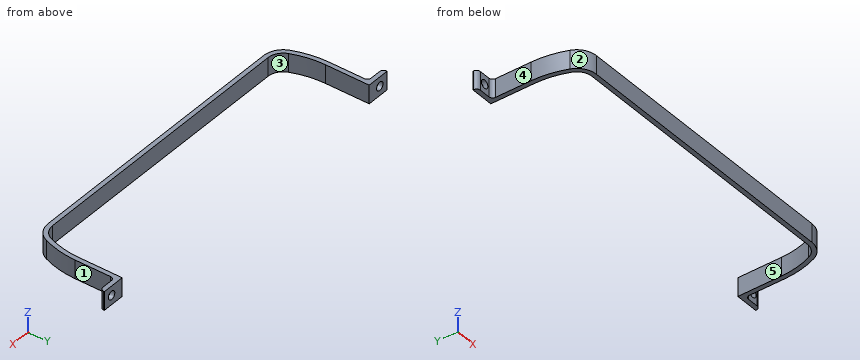
from build123d import *

# Parameters (mm, degrees)
F1_DEPTH = 5
F3_D     = 4.4958
F4_R     = 2


with BuildPart() as f1:
    # F0 (on Top) → F1 (new body, symmetric)
    with BuildSketch(Plane.XY):
        with BuildLine():
            Line((0, 2.4), (0, 0))
            Line((0, 0), (75, 0))
            ThreePointArc((75, 0), (80.9415780593, 1.816522709), (84.8515829028, 6.6449765723))
            ThreePointArc((84.8515829028, 6.6449765723), (87.5046708667, 15.6016514337), (88.4, 24.9))
            Line((88.4, 24.9), (88.4, 46))
            Line((88.4, 46), (98.4, 46))
            Line((98.4, 46), (98.4, 48.4))
            Line((98.4, 48.4), (86, 48.4))
            Line((86, 48.4), (86, 24.9))
            ThreePointArc((86, 24.9), (85.1487656265, 16.0595930226), (82.6263416519, 7.5440323965))
            ThreePointArc((82.6263416519, 7.5440323965), (79.5995150909, 3.8062128831), (75, 2.4))
            Line((75, 2.4), (0, 2.4))
        make_face()
    extrude(amount=F1_DEPTH, both=True)

    # F3 (through all)
    with Locations(Plane.XZ.offset(-46)):
        with Locations((93.4, 0)):
            Hole(F3_D / 2)

    # F4
    f4_edges = [f1.edges().sort_by_distance(p)[0] for p in [
        (88.4, 46, 0),
        (98.4, 46, 0),
    ]]
    fillet(f4_edges, radius=F4_R)

    # F5: F1 across face


with BuildPart() as f1_1:
    add(f1.part)
    add(f1.part.mirror(Plane(origin=(0, 1.2, 0), x_dir=(0, -1, 0), z_dir=(-1, 0, 0))))


solid = f1_1.part
Design review of the part built by this model. Coordinates are the model's own, in mm. Face numbers are marked on the shaded views. A direction names the side the tool comes from. Coordinates: 2 decimals unless noted, no trailing zeros. Write each loop counter-clockwise with the first axis right and the second up, starting at its lowest first coordinate (ties: lowest second). Pieces come first, ordered by that corner, then holes. Notation, with made-up numbers: (-32.5, 77) -> (14.5, 77) arc R23 cw to (14.5, 107) -> close; hole circle Ø1 at (-10, 44.5). An arc over 180 degrees is marked (long way). Write each question's results on one line, items separated by ' | '. Start each with the question number.
(1) For line 1 along Z through (x, y) = (-93.4, 47.2); line 2 along X through (y, z) = (39.5, -2); line 3 along Y through (x, z) = (-34.5, 0.75), list the stretches that pass through material, from the lowest coordinate up. Write a range as from..to.
(2) Take a section at C-C on y = 14. Write out the cut boundary in (x, z), and give its area (3 significant figures).
(3) The part is to be moulded in two halves that separate along X. For the marked faces 1, 2 and 3, say which applies: pulls with the +X half, pulls with the -X half, needs draft (parallel to the pull), parting line crosses it, or undercut.
(4) Clearance check with flat-ended pins moving along their axes: P1, Ø3, axis at x = -92.5, z = 0.5, coming from the -Y side; P2, Ø3, axis at y = 34, z = -1.5, coming from the +X side; P3, Ø1.5, axis at x = -72, z = 0.5, coming from the +Y side. State where each tip first meets the part, or that it passes through.
(5) Take a section at A-A on z = 0. Give the number of separate pieces and of enclosed holes in the cut face, and give its area (3 significant figures).
(6) Take a section at D-D on x = 24.5. Write out the cut boundary in (y, z).
(7) Tool access review of the marked faces 4 and 5: name each direction out of +Z, -Z, +X, -X, +Y, -Y from which nothing blocks a thin tool from reaching the whole face with its end or side.
(8) Take a section at B-B on x = 93.4. Write out the cut boundary in (y, z), and give its area (3 significant figures).
Results found:
1) line 1: z = -5..-2.25, 2.25..5 | line 2: x = -88.4..-86, 86..88.4 | line 3: y = 0..2.4
2) outline: (-87.17, -5) -> (-84.7, -5) -> (-84.7, 5) -> (-87.17, 5) -> close; (84.7, -5) -> (87.17, -5) -> (87.17, 5) -> (84.7, 5) -> close | area: 49.3 mm2
3) face 1: pulls with the +X half | face 2: pulls with the -X half | face 3: undercut
4) P1: stops at y = 46 | P2: stops at x = 88.4 | P3: stops at y = 2.4
5) separate pieces: 3 | enclosed holes: 0 | area: 641 mm2
6) outline: (0, -5) -> (2.4, -5) -> (2.4, 5) -> (0, 5) -> close
7) face 4: +Z, -Z, -X, -Y | face 5: +Z, -Z, +Y
8) outline: (46, -5) -> (48.4, -5) -> (48.4, -2.25) -> (46, -2.25) -> close; (46, 2.25) -> (48.4, 2.25) -> (48.4, 5) -> (46, 5) -> close | area: 13.2 mm2
